Drawing for the job (mm, zero at the part's lowest x, y, z). Round coordinates to 2 decimals unless told otherwise and drop trailing zeros. Loops run counter-clockwise (first coordinate to the right, second up) from the corner with the lowest first, then second, coordinate; pieces in that order, holes last. Notation, with made-up numbers: (41, 46.25) - (48, 46.25) arc R5 ccw to (48, 54.25) - close; hole circle Ø2 at (15.5, 34). An arc over 180 degrees is marked (long way). Put each result on its own line as item: value.
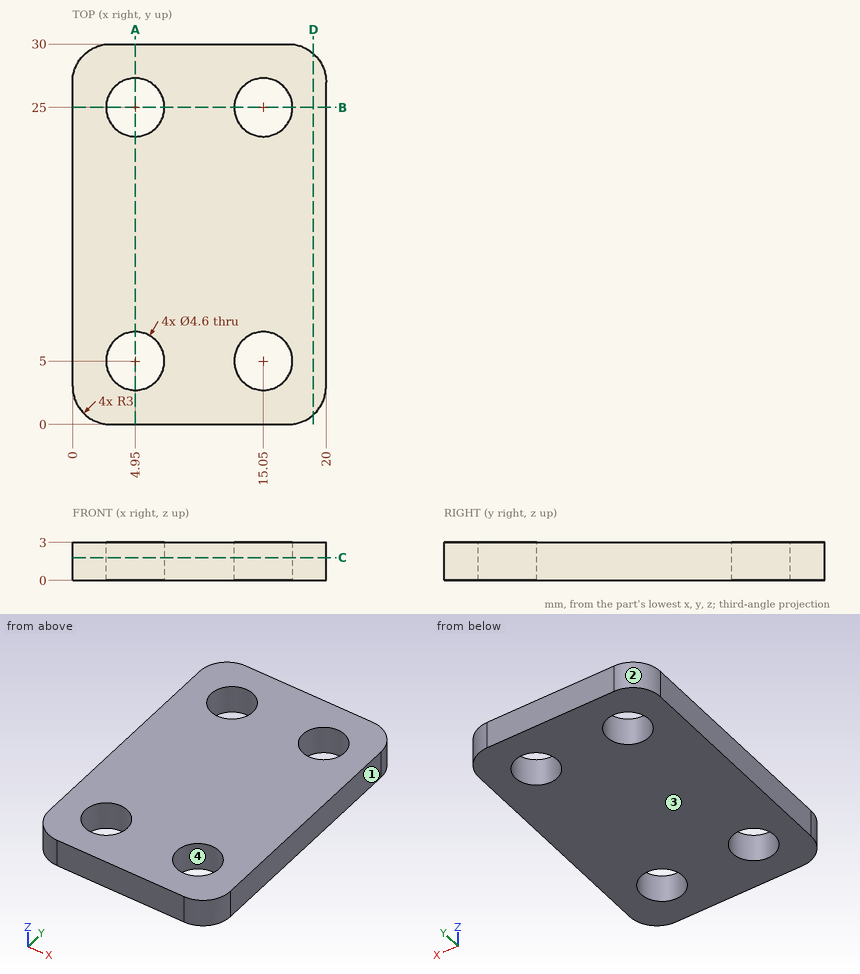
1. Band-saw the part on A-A (x = 4.95). List the corners of the cut face in (y, z), plus the area to 3 significant figures.
A:
outline: (0, 0) - (2.7, 0) - (2.7, 3) - (0, 3) - close; (7.3, 0) - (22.7, 0) - (22.7, 3) - (7.3, 3) - close; (27.3, 0) - (30, 0) - (30, 3) - (27.3, 3) - close
area: 62.4 mm²
2. Band-saw the part on B-B (y = 25). List the corners of the cut face in (x, z).
A:
outline: (0, 0) - (2.65, 0) - (2.65, 3) - (0, 3) - close; (7.25, 0) - (12.75, 0) - (12.75, 3) - (7.25, 3) - close; (17.35, 0) - (20, 0) - (20, 3) - (17.35, 3) - close
3. Two-plate mould, pull along X, no slides. Class the marked faces 1, 2, 3 and 4: pulls with the +X half, pulls with the -X half, needs draft (parallel to the pull), parting line crosses it, or undercut.
A:
face 1: pulls with the +X half
face 2: pulls with the -X half
face 3: needs draft
face 4: undercut
4. Pin check, flat tips, straight feed: P1, Ø6, axis at x = 15.05, y = 5, coming from the -Z side; P2, Ø4, axis at x = 15.05, y = 25, coming from the +Z side. Stop position of each tip, or through.
A:
P1: stops at z = 0
P2: passes through
5. Band-saw the part on D-D (x = 19). List the corners of the cut face in (y, z), plus the area to 3 significant figures.
A:
outline: (0.76, 0) - (29.24, 0) - (29.24, 3) - (0.76, 3) - close
area: 85.4 mm²
6. Probe line 1 along Y through (x, z) = (15.05, 1.55); line 2 along Y through (x, z) = (3, 0.5); line 3 along X through (y, z) = (23, 1.95). List the from-to ranges inside material, lowest first. Write a range as [from, to].
A:
line 1: y = [0, 2.7], [7.3, 22.7], [27.3, 30]
line 2: y = [0, 3.78], [6.22, 23.78], [26.22, 30]
line 3: x = [0, 3.81], [6.09, 13.91], [16.19, 20]
7. Band-saw the part on C-C (z = 1.8). List the corners of the cut face in (x, y).
A:
outline: (0, 3) arc R3 ccw to (3, 0) - (17, 0) arc R3 ccw to (20, 3) - (20, 27) arc R3 ccw to (17, 30) - (3, 30) arc R3 ccw to (0, 27) - close; hole circle Ø4.6 at (4.95, 5); hole circle Ø4.6 at (4.95, 25); hole circle Ø4.6 at (15.05, 5); hole circle Ø4.6 at (15.05, 25)
